Verification items for the finished model (mm, model axes). A direction names the side the tool comes from. Give positions to 0.01 mm unless a question says otherwise; leave off trailing zeros. Write each loop counter-clockwise with the first axis right and the second up, starting at its lowest first coordinate (ties: lowest second). Pieces come first, ordered by that corner, then holes. Notation, with made-up numbers: (61.5, 6) - (88.5, 6) arc R22 ccw to (88.5, 42) - close; hole circle Ø1 at (87, 89). An arc over 180 degrees is marked (long way). Answer as a JSON object with one key per item and string values. Group by question number.
Item 1: Tool access check on faces 1 (the face through (64, 16, 1)), 2 (the face through (41, 82, 1)), 3 (the face through (66, 19, 1)). Record the directions out of +Z, -Z, +X, -X, +Y, -Y that give a thin tool (end or side, any length) a straight path to the whole face; none if there is none.
Item 2: Sectioned sample at B-B, the plane y = 56. Record the boundary of the cut face in (x, z), and give its area (4 significant figures).
Item 3: Scan lines: line 1 along Y through (x, z) = (46, 2.4); line 2 along Y through (x, z) = (41.5, 1.9); line 3 along X through (y, z) = (88, 1.4). Record each from-to range of solid material in increasing order. Write a range as [from, to].
Item 4: Go/stop test with flat-tipped pins: pin 1 (1.5 mm diameter, centred on y = 76, z = 2, fed in from +X); pin 2 (1.5 mm diameter, centred on y = 120.5, z = 1, fed in from -X). Record where each tip stops, or that it passes through.
Item 5: Draft check along X on faces 4 (the face through (57, 36, 1)), 5 (the face through (53, 38, 1)), 6 (the face through (63, 3, 1)). Enter one of: +X half, -X half, draft (parallel to the pull), parting line (faces both ways), or undercut.
Item 6: Sectioned sample at A-A, the plane x = 64.5. Count the separate pieces of the cut face and the enclosed holes in it, and give its area (3 significant figures).
```python
from build123d import *

# Parameters (mm, degrees)
SKETCH_1_W      = 8
SKETCH_1_H      = 3
EXTRUDE_1_DEPTH = 3


with BuildPart() as part:
    # 草图1 → 凸台-拉伸1 (new body)
    with BuildSketch(Plane.XY):
        with BuildLine():
            Line((63, 10), (63, 16))
            Line((63, 16), (66, 16))
            Line((66, 16), (66, 22.677124344))
            ThreePointArc((66, 22.677124344), (62.5, 24), (66, 25.322875656))
            Line((66, 25.322875656), (66, 32))
            Line((66, 32), (63, 32))
            Line((63, 32), (63, 38))
            Line((63, 38), (58, 38))
            Line((58, 38), (58, 36))
            Line((58, 36), (55, 36))
            Line((55, 36), (55, 38))
            Line((55, 38), (51, 38))
            Line((51, 38), (51, 42))
            Line((51, 42), (55, 42))
            Line((55, 42), (55, 44))
            Line((55, 44), (58, 44))
            Line((58, 44), (58, 42))
            Line((58, 42), (63, 42))
            Line((63, 42), (63, 48))
            Line((63, 48), (66, 48))
            Line((66, 48), (66, 54.677124344))
            ThreePointArc((66, 54.677124344), (62.5, 56), (66, 57.322875656))
            Line((66, 57.322875656), (66, 64))
            Line((66, 64), (63, 64))
            Line((63, 64), (63, 70))
            Line((63, 70), (58, 70))
            Line((58, 70), (58, 68))
            Line((58, 68), (55, 68))
            Line((55, 68), (55, 70))
            Line((55, 70), (51, 70))
            Line((51, 70), (51, 74))
            Line((51, 74), (55, 74))
            Line((55, 74), (55, 76))
            Line((55, 76), (58, 76))
            Line((58, 76), (58, 74))
            Line((58, 74), (63, 74))
            Line((63, 74), (63, 80))
            Line((63, 80), (66, 80))
            Line((66, 80), (66, 86.677124344))
            ThreePointArc((66, 86.677124344), (62.5, 88), (66, 89.322875656))
            Line((66, 89.322875656), (66, 96))
            Line((66, 96), (63, 96))
            Line((63, 96), (63, 129))
            Line((63, 129), (0, 129))
            Line((0, 129), (0, 0))
            Line((0, 0), (0, -16))
            Line((0, -16), (66, -16))
            Line((66, -16), (66, -9.322875656))
            ThreePointArc((66, -9.322875656), (62.5, -8), (66, -6.677124344))
            Line((66, -6.677124344), (66, 0))
            Line((66, 0), (63, 0))
            Line((63, 0), (63, 6))
            Line((63, 6), (58, 6))
            Line((58, 6), (58, 4))
            Line((58, 4), (55, 4))
            Line((55, 4), (55, 6))
            Line((55, 6), (51, 6))
            Line((51, 6), (51, 10))
            Line((51, 10), (55, 10))
            Line((55, 10), (55, 12))
            Line((55, 12), (58, 12))
            Line((58, 12), (58, 10))
            Line((58, 10), (63, 10))
        make_face()
        with Locations((39, 2.5)):
            Rectangle(SKETCH_1_W, SKETCH_1_H, mode=Mode.SUBTRACT)
        with Locations((39, 65.5)):
            Rectangle(SKETCH_1_W, SKETCH_1_H, mode=Mode.SUBTRACT)
        Polygon((47, 89), (47, 84), (47, 79), (44, 79), (44, 84), (41, 84), (41, 79), (38, 79), (38, 84), (35, 84), (35, 79), (32, 79), (32, 84), (29, 84), (29, 79), (26, 79), (26, 89), (32, 89), align=None, mode=Mode.SUBTRACT)
        Polygon((5, 114), (5, 124), (8, 124), (8, 119), (11, 119), (11, 124), (14, 124), (14, 119), (17, 119), (17, 124), (20, 124), (20, 119), (23, 119), (23, 124), (26, 124), (26, 119), (29, 119), (29, 124), (32, 124), (32, 119), (35, 119), (35, 124), (38, 124), (38, 119), (41, 119), (41, 124), (44, 124), (44, 119), (47, 119), (47, 124), (50, 124), (50, 114), align=None, mode=Mode.SUBTRACT)
    extrude(amount=EXTRUDE_1_DEPTH)


solid = part.part
```
Geometry check:
{
 "1": {"face 1": "+Z, -Z, +X", "face 2": "+Z, -Z", "face 3": "+Z, -Z, +X, +Y, -Y"},
 "2": {"outline": "(0, 0) - (62.5, 0) - (62.5, 3) - (0, 3) - close", "area": "187.5 mm^2"},
 "3": {"line 1": "[-16, 79], [89, 114], [119, 129]", "line 2": "[-16, 1], [4, 64], [67, 84], [89, 114], [124, 129]", "line 3": "[0, 26], [47, 62.5]"},
 "4": {"pin 1": "x = 63", "pin 2": "x = 0"},
 "5": {"face 4": "undercut", "face 5": "draft", "face 6": "+X half"},
 "6": {"separate pieces": "8", "enclosed holes": "0", "area": "144 mm^2"}
}
